```python
from build123d import *

# Parameters (mm, degrees)
BOSS_EXTRUDE1_DEPTH = 75
SKETCH2_W           = 42
SKETCH2_H           = 40
SKETCH2_R           = 2.5
BOSS_EXTRUDE2_DEPTH = 4
BOSS_EXTRUDE3_DEPTH = 3
SKETCH4_R           = 2.5
CUT_EXTRUDE1_DEPTH  = 3
SKETCH5_W           = 43
SKETCH5_H           = 16.5
SKETCH5_R           = 4
BOSS_EXTRUDE4_DEPTH = 45
SKETCH6_W           = 45
SKETCH6_H           = 20.5
BOSS_EXTRUDE6_DEPTH = 3


with BuildPart() as part:
    # Sketch1 → Boss-Extrude1 (new body)
    with BuildSketch(Plane(origin=(0, 0, 0), x_dir=(1, 0, 0), z_dir=(0, 1, 0))):
        Polygon((0, 0), (0, 40), (3, 40), (3, -3), (-22, -3), (-22, 0), align=None)
    extrude(amount=BOSS_EXTRUDE1_DEPTH)

    # Sketch2 → Boss-Extrude2 (add)
    with BuildSketch(Plane(origin=(0, 75, 0), x_dir=(1, 0, 0), z_dir=(0, 1, 0))):
        with Locations((-21, 20)):
            Rectangle(SKETCH2_W, SKETCH2_H)
        with Locations(Location((-17, 20, 0), (0, 0, 270))):
            Circle(SKETCH2_R, mode=Mode.SUBTRACT)
    extrude(amount=-BOSS_EXTRUDE2_DEPTH)

    # Sketch3 → Boss-Extrude3 (add)
    with BuildSketch(Plane.XY):
        Polygon((-22, 75), (-42, 75), (-42, 71), (-22, 51), align=None)
    extrude(amount=BOSS_EXTRUDE3_DEPTH)

    # Sketch4 → Cut-Extrude1 (cut)
    with BuildSketch(Plane(origin=(3, 0, 0), x_dir=(0, 0, -1), z_dir=(1, 0, 0))):
        with Locations((18.5, 25)):
            Circle(SKETCH4_R)
    extrude(amount=-CUT_EXTRUDE1_DEPTH, mode=Mode.SUBTRACT)

    # Sketch5 → Boss-Extrude4 (add)
    with BuildSketch(Plane.ZY.offset(42)):
        with Locations((-18.5, 83.25)):
            Rectangle(SKETCH5_W, SKETCH5_H)
        with Locations((-35, 83.5)):
            Circle(SKETCH5_R, mode=Mode.SUBTRACT)
        with Locations((-5, 83.5)):
            Circle(SKETCH5_R, mode=Mode.SUBTRACT)
    extrude(amount=-BOSS_EXTRUDE4_DEPTH)

    # Sketch6 → Boss-Extrude6 (add)
    with BuildSketch(Plane(origin=(0, 0, -40), x_dir=(-1, 0, 0), z_dir=(0, 0, -1))):
        with Locations((19.5, 81.25)):
            Rectangle(SKETCH6_W, SKETCH6_H)
    extrude(amount=BOSS_EXTRUDE6_DEPTH)


solid = part.part
```
Can you work these out from the model? Positions are in its coordinate system, mm. A direction names the side the tool comes from. Round coordinates to 2 decimals unless told otherwise and drop trailing zeros. Loops run counter-clockwise (first coordinate to the right, second up) from the corner with the lowest first, then second, coordinate; pieces in that order, holes last. Notation, with made-up numbers: M 9.5,4.5 L 59.5,4.5 A21 cw 59.5,20.5 Z; hole C 14.25,68.5 d3. An arc over 180 degrees is marked long. Answer as a JSON object with one key per item and string values. Group by question number.
Q1. On a 3-axis mill with a long thin cutter (end or side, diameter ignored), from which of +Z, -Z, +X, -X, +Y, -Y can I reach the whole of each face in a straight line? I mean faces 1 (the flat face through (0, 35, -20)), 2 (the cylindrical face through (-16.9, 73, -22.5)), 3 (the cylindrical face through (-19.815, 79.595, -5.867)). Say none if no direction works.
Q2. Imagine slicing it at B-B, the plane z = -20. Please give me the cut outline in (x, y).
Q3. Imagine slicing it at D-D, the plane y = 25. Please give me the cut outline in (x, z).
Q4. Imagine slicing it at A-A, the plane y = 83.5. Please give me the cut outline in (x, z), then the cut area to 3 significant figures.
Q5. Will these pins go through, and if not, where does the flat tip stop? pin 1 (5 mm diameter, centred on x = -4, y = 47.5, fed in from -Z); pin 2 (4 mm diameter, centred on x = -17, z = -20, fed in from -Y); pin 3 (9 mm diameter, centred on y = 83.5, z = -35, fed in from -X); pin 4 (10 mm diameter, centred on y = 48.5, z = -2, fed in from -X).
Q6. We'd pull the mould along X, two halves only. Please class faces 4 (the flat face through (-17, 75, -20)), 5 (the flat face through (3, 45, -20)), 6 (the flat face through (1, 35, -40)), 7 (the flat face through (-22, 25, 2)): +X half, -X half, draft (parallel to the pull), parting line (faces both ways), or undercut.
Q7. Please list where these lines run through material, in increasing order: L1, parallel to Y at x = 1.3, z = -18.5; L2, parallel to Y at x = -3, z = -35; L3, parallel to X at y = 73, z = -20.
Q8. Imagine slicing it at C-C, the plane x = -17. Please give me the cut outline in (y, z).
Findings:
{
 "1": {"face 1": "-Z, -X, -Y", "face 2": "-Y", "face 3": "+X, -X"},
 "2": {"outline": "M -42,71 L -19.5,71 L -19.5,75 L -14.5,75 L -14.5,71 L 0,71 L 0,27 L 3,27 L 3,91.5 L -42,91.5 Z; M 0,0 L 3,0 L 3,23 L 0,23 Z"},
 "3": {"outline": "M -22,0 L 0,0 L 0,-16 L 3,-16 L 3,3 L -22,3 Z; M 0,-40 L 3,-40 L 3,-21 L 0,-21 Z"},
 "4": {"outline": "M -42,-43 L 3,-43 L 3,-39 L -42,-39 Z; M -42,-31 L 3,-31 L 3,-9 L -42,-9 Z; M -42,-1 L 3,-1 L 3,3 L -42,3 Z", "area": "1,350 mm2"},
 "5": {"pin 1": "stops at z = 0", "pin 2": "stops at y = 75", "pin 3": "stops at x = -42", "pin 4": "stops at x = -24.08"},
 "6": {"face 4": "undercut", "face 5": "+X half", "face 6": "draft", "face 7": "-X half"},
 "7": {"L1": "y = 0 to 22.5, 27.5 to 91.5", "L2": "y = 71 to 79.5, 87.5 to 91.5", "L3": "x = -42 to -19.5, -14.5 to 3"},
 "8": {"outline": "M 0,0 L 71,0 L 71,-17.5 L 75,-17.5 L 75,-22.5 L 71,-22.5 L 71,-43 L 91.5,-43 L 91.5,3 L 0,3 Z; hole C 83.5,-35 d8; hole C 83.5,-5 d8"}
}
